Geometry: final body of the model. Coordinates: model frame, mm. Face numbers are marked on the shaded views. Round coordinates to 2 decimals unless told otherwise and drop trailing zeros. Order: outer loops, then holes, each group sorted by start corner. A loop starts at its lowest first (then second) coordinate and runs counter-clockwise, first axis right, second up. Notation, with made-up numbers: (20.5, 38.5) - (24.5, 38.5) arc R19 ccw to (24.5, 68.5) - close; hole circle Ø11 at (-3.5, 59.25). An arc over 180 degrees is marked (long way). Put each result on its own line as item: value. Start each with the question number.
(1) Section B-B (y = 13). Output: boundary loops of the cut face in (x, z).
(2) Section C-C (x = 121.5). Output: boundary loops of the cut face in (y, z).
(3) Section A-A (z = 1.1). Count the separate pieces of the cut face and the enclosed holes in it, and give its area (3 significant figures).
(4) Pull-direction query (Z, two-part tool) for the marked faces 1 and 2; classes: released by +Z, released by -Z, zero draft, split by the parting line, or undercut.
(5) Pin query (flat end, axial travel): P1, Ø2, axis at x = 139.5, z = 3, coming from the -Y side; P2, Ø1.5, axis at y = 8.5, z = 1.5, coming from the -X side; P3, Ø1.8, axis at y = 17, z = 3.5, coming from the -X side. Return the tip coordinate at first contact, or that it passes through.
(6) Material intervals for L1, parallel to Y at x = 26, z = 3.85; L2, parallel to X at y = -2, z = 0.35; L3, parallel to X at y = 18, z = 3.55, sorted ascending. Write a range as [from, to].
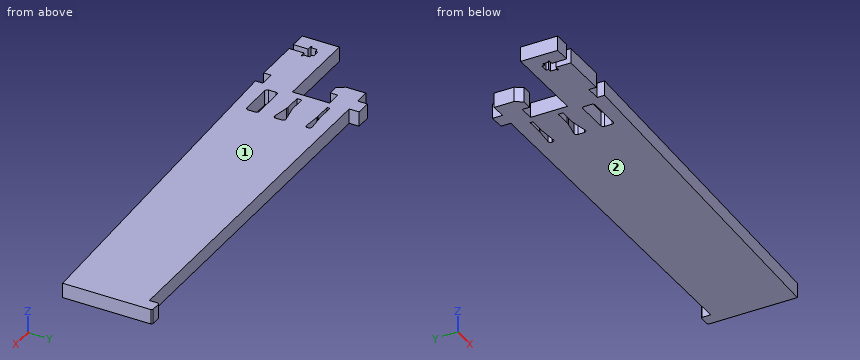
from build123d import *

# Parameters (mm, degrees)
SKETCH1_W           = 15
SKETCH1_H           = 5
BOSS_EXTRUDE1_DEPTH = 6
CHAMFER1_SIZE       = 3
CHAMFER1_SIZE2      = 2
FILLET1_R           = 1
FILLET2_R           = 5
CHAMFER2_SIZE       = 0.5


with BuildPart() as part:
    # Sketch1 → Boss-Extrude1 (new body)
    with BuildSketch(Plane.XY):
        Polygon((-17.5, -7), (16.5, -7), (16.5, 8), (10.5, 8), (10.5, 5), (4.5, 5), (4.5, 16), (10.5, 16), (10.5, 20), (16.5, 20), (16.5, 16), (161.5, 16), (161.5, 20), (166.5, 20), (166.5, -16.342859565), (16.5, -22), (16.5, -19), (10.5, -19), (10.5, -22), (-8.02, -22), (-8.02, -16), (-6, -16), (-6, -15.5), (-6.75, -15.5), (-6.75, -13), (-8.02, -13), (-8.02, -12), (-10.98, -12), (-10.98, -13), (-12.25, -13), (-12.25, -15.5), (-13, -15.5), (-13, -16), (-10.98, -16), (-10.98, -22), (-17.5, -22), align=None)
        Polygon((19.5, -3.45), (19.5, -1.55), (26.5, -1.55), (34.5, 0), (34.5, -5), (26.5, -3.45), align=None, mode=Mode.SUBTRACT)
        with Locations((27, -13.5)):
            Rectangle(SKETCH1_W, SKETCH1_H, mode=Mode.SUBTRACT)
        Polygon((19.5, 8.726722117), (19.5, 9.826722117), (26.5, 9.826722117), (34.5, 10.487607038), (34.5, 8.065837195), (26.5, 8.726722117), align=None, mode=Mode.SUBTRACT)
    extrude(amount=BOSS_EXTRUDE1_DEPTH)

    # Chamfer1
    chamfer1_edges = [part.edges().sort_by_distance(p)[0] for p in [
        (4.5, 5, 3),
    ]]
    chamfer1_side = [part.faces().sort_by_distance(p)[0] for p in [
        (4.5, 10.5, 3),
    ]]
    chamfer(chamfer1_edges, length=CHAMFER1_SIZE, length2=CHAMFER1_SIZE2, reference=chamfer1_side[0])

    # Fillet1
    fillet1_edges = [part.edges().sort_by_distance(p)[0] for p in [
        (19.5, -16, 3),
        (34.5, -16, 3),
        (34.5, -11, 3),
        (19.5, -11, 3),
        (34.5, 8.065837195, 3),
        (34.5, 10.487607038, 3),
        (34.5, -5, 3),
        (34.5, 0, 3),
    ]]
    fillet(fillet1_edges, radius=FILLET1_R)

    # Fillet2
    # the kernel refuses this fillet: 5 mm, written as the material it takes off along each edge
    with BuildSketch(Plane(origin=(26.5, 8.726722117, -0.515438436), x_dir=(0.9966051096378002, -0.08233016120370525, 0), z_dir=(0, 0, 1)), Plane(origin=(26.5, 9.826722117, -0.515438436), x_dir=(-1, 0, 0), z_dir=(0, 0, 1))) as fillet2_piece_1:
        with BuildLine():
            CenterArc((FILLET2_R * 0.041235074881, -FILLET2_R), FILLET2_R, 90, 4.722516116)
            Line((-FILLET2_R * 0.0410950863227, -FILLET2_R * 0.0033948903622), (0, 0))
            Line((0, 0), (FILLET2_R * 0.041235074881, 0))
        make_face()
    extrude(amount=7.030876872, mode=Mode.SUBTRACT)
    with BuildSketch(Plane(origin=(26.5, -3.45, -1.199781563), x_dir=(0.9817429059156794, -0.19021268802116595, 0), z_dir=(0, 0, 1)), Plane(origin=(26.5, -1.55, -1.199781563), x_dir=(-1, 0, 0), z_dir=(0, 0, 1))) as fillet2_piece_2:
        with BuildLine():
            CenterArc((FILLET2_R * 0.0959825250053, -FILLET2_R), FILLET2_R, 90, 10.965196685)
            Line((-FILLET2_R * 0.0942301630158, -FILLET2_R * 0.0182570940843), (0, 0))
            Line((0, 0), (FILLET2_R * 0.0959825250053, 0))
        make_face()
    extrude(amount=8.399563125, mode=Mode.SUBTRACT)

    # Chamfer2
    chamfer2_edges = [part.edges().sort_by_distance(p)[0] for p in [
        (161.5, 20, 3),
        (166.5, 20, 3),
    ]]
    chamfer(chamfer2_edges, length=CHAMFER2_SIZE)


solid = part.part
Checks:
1. outline: (4.5, 0) - (166.5, 0) - (166.5, 6) - (4.5, 6) - close
2. outline: (-18.04, 0) - (16, 0) - (16, 6) - (-18.04, 6) - close
3. separate pieces: 1
3. enclosed holes: 3
3. area: 5,750 mm²
4. face 1: released by +Z
4. face 2: released by -Z
5. P1: stops at y = -17.4
5. P2: stops at x = 4.5
5. P3: stops at x = 10.5
6. L1: y = [-21.64, -16], [-11, -3.45], [-1.55, 8.73], [9.83, 16]
6. L2: x = [16.5, 19.5], [34.5, 166.5]
6. L3: x = [10.5, 16.5], [161.5, 166.5]
